Drawing for the job (mm, zero at the part's lowest x, y, z). A direction names the side the tool comes from. Give positions to 0.01 mm unless a question says otherwise; leave off trailing zeros. Write each loop counter-clockwise with the first axis right and the second up, starting at its lowest first coordinate (ties: lowest second). Pieces come first, ordered by that corner, then holes. Notation, with made-up numbers: M 68,89 L 80,89 A28 cw 80,116 Z; hole C 87,49.25 d3. An arc over 180 degrees is marked long. Write item = value, one per line. Start each with the question number.
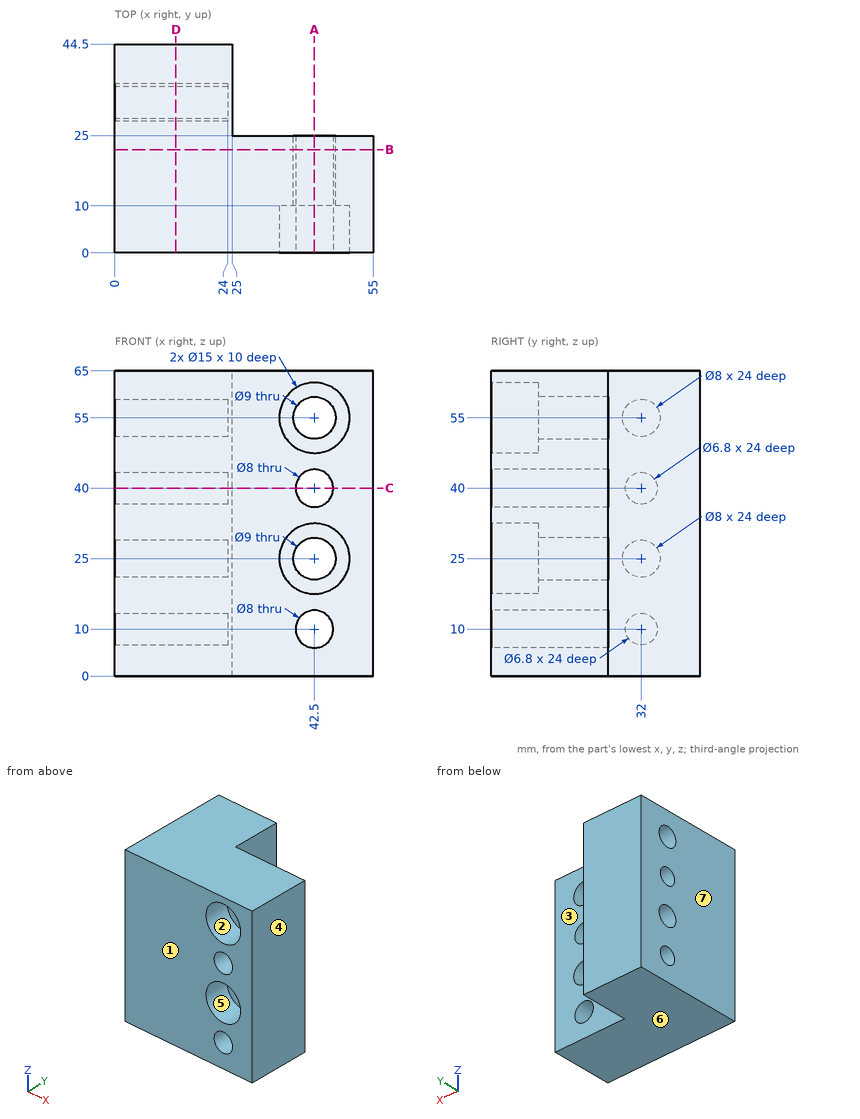
Q1. Slice it at D-D (x = 13). Give the cut face in (y, z).
Q2. Two-plate mould, pull along X, no slides. Class the marked faces 4, 5, 6 and 7: +X half, -X half, draft (parallel to the pull), parting line (faces both ways), or undercut.
Q3. Slice it at C-C (z = 40). Give the cut face in (x, y).
Q4. Drop flat-ended pins along their axis: P1, Ø6.5, axis at y = 31.5, z = 54, coming from the -X side; P2, Ø7, axis at x = 42.5, z = 25, coming from the -Y side; P3, Ø13.5, axis at x = 42.5, z = 55, coming from the -Y side; P4, Ø11.5, axis at x = 42.5, z = 55, coming from the +Y side. Give the stop position or say it passes through.
Q5. Tool access for the marked faces 1, 2 and 3: list every direction of +Z, -Z, +X, -X, +Y, -Y with a clear straight run to the whole face (end or side of a thin tool).
Q6. Probe line 1 along X through (y, z) = (22, 55); line 2 along Z through (x, y) = (42, 2); line 3 along Y through (x, z) = (15, 55). List the from-to ranges inside material, lowest first.
Q7. Slice it at B-B (y = 22). Give the cut face in (x, z), and give its area (3 significant figures).
Q8. Slice it at A-A (x = 42.5). Give the cut face in (y, z), and give its area (3 significant figures).
Working result:
q1.outline = M 0,0 L 44.5,0 L 44.5,65 L 0,65 Z; hole C 32,25 d8; hole C 32,55 d8; hole C 32,10 d6.8; hole C 32,40 d6.8
q2.face_4 = +X half
q2.face_5 = undercut
q2.face_6 = draft
q2.face_7 = -X half
q3.outline = M 0,0 L 38.5,0 L 38.5,25 L 25,25 L 25,44.5 L 0,44.5 L 0,35.4 L 24,35.4 L 24,28.6 L 0,28.6 Z; M 46.5,0 L 55,0 L 55,25 L 46.5,25 Z
q4.P1 = 0
q4.P2 = through
q4.P3 = 10
q4.P4 = 25
q5.face_1 = +Z, -Z, +X, -X, -Y
q5.face_2 = -Y
q5.face_3 = +Z, -Z, +X, +Y
q6.line_1 = 0 to 38, 47 to 55
q6.line_2 = 0 to 6.03, 13.97 to 17.52, 32.48 to 36.03, 43.97 to 47.52, 62.48 to 65
q6.line_3 = 0 to 28, 36 to 44.5
q7.outline = M 0,0 L 55,0 L 55,65 L 0,65 Z; hole C 42.5,25 d9; hole C 42.5,55 d9; hole C 42.5,10 d8; hole C 42.5,40 d8
q7.area = 3,350 mm2
q8.outline = M 0,0 L 25,0 L 25,6 L 0,6 Z; M 0,14 L 25,14 L 25,20.5 L 10,20.5 L 10,17.5 L 0,17.5 Z; M 0,32.5 L 10,32.5 L 10,29.5 L 25,29.5 L 25,36 L 0,36 Z; M 0,44 L 25,44 L 25,50.5 L 10,50.5 L 10,47.5 L 0,47.5 Z; M 0,62.5 L 10,62.5 L 10,59.5 L 25,59.5 L 25,65 L 0,65 Z
q8.area = 655 mm2
